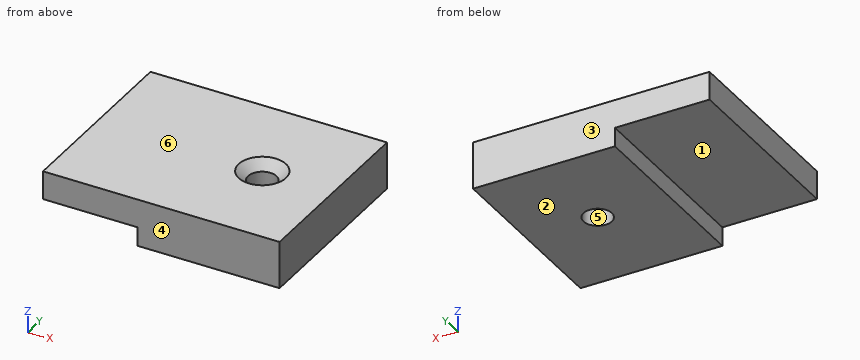
```python
from build123d import *

# Parameters (mm, degrees)
F1_DEPTH = 20
F2_R     = 1.5
F3_DEPTH = 5.001
F4_SIZE  = 1


with BuildPart() as f1:
    # F0 (on Front) → F1 (new body)
    with BuildSketch(Plane.XZ):
        Polygon((-22.628114, -7.176122), (-12.628114, -7.176122), (-12.628114, -9.176122), (2.371886, -9.176122), (2.371886, -4.176122), (-22.628114, -4.176122), align=None)
    extrude(amount=F1_DEPTH)

    # F2 (on face) → F3 (cut, through all)
    with BuildSketch(Plane(origin=(0, 0, -9.176122), x_dir=(1, 0, 0), z_dir=(0, 0, -1))):
        with Locations((-5.128114, 10)):
            Circle(F2_R)
    extrude(amount=-F3_DEPTH, mode=Mode.SUBTRACT)

    # F4
    f4_edges = [f1.edges().sort_by_distance(p)[0] for p in [
        (-6.628114, -10, -4.176122),
    ]]
    chamfer(f4_edges, length=F4_SIZE)


solid = f1.part
```
The model under review builds one solid part; all positions refer to its coordinate system, in mm. Face numbers are marked on the shaded views. A direction names the side the tool comes from. Give positions to 0.01 mm unless a question says otherwise; leave off trailing zeros. Write each loop counter-clockwise with the first axis right and the second up, starting at its lowest first coordinate (ties: lowest second). Pieces come first, ordered by that corner, then holes. Notation, with made-up numbers: M -11,23 L 30,23 A22 ccw 30,38 Z; hole C 85,19 d1. An arc over 180 degrees is marked long. Answer in a Markdown table with one row per item.
Item 1: Draft analysis for pull direction Y (two halves, no side actions). For the marked faces 3, 4, 5 and 6, state which applies: +Y half, -Y half, draft (parallel to the pull), parting line (faces both ways), or undercut.
Check sheet entries:
| item | result |
|---|---|
| face 3 | +Y half |
| face 4 | -Y half |
| face 5 | undercut |
| face 6 | draft |
Item 2: Add section A-A on y = -10. Give the boundary of the cut face in (x, z).
Check sheet entries:
| item | result |
|---|---|
| outline | M -22.63,-7.18 L -12.63,-7.18 L -12.63,-9.18 L -6.63,-9.18 L -6.63,-5.18 L -7.63,-4.18 L -22.63,-4.18 Z; M -3.63,-9.18 L 2.37,-9.18 L 2.37,-4.18 L -2.63,-4.18 L -3.63,-5.18 Z |
Item 3: Add section B-B on y = -4.75. Give the boundary of the cut face in (x, z), plus the area to 3 significant figures.
Check sheet entries:
| item | result |
|---|---|
| outline | M -22.63,-7.18 L -12.63,-7.18 L -12.63,-9.18 L 2.37,-9.18 L 2.37,-4.18 L -22.63,-4.18 Z |
| area | 105 mm2 |
Item 4: Add section D-D on x = -16.25. Give the boundary of the cut face in (y, z).
Check sheet entries:
| item | result |
|---|---|
| outline | M -20,-7.18 L 0,-7.18 L 0,-4.18 L -20,-4.18 Z |
Item 5: Tool access review of the marked faces 1 and 2: name each direction out of +Z, -Z, +X, -X, +Y, -Y from which nothing blocks a thin tool from reaching the whole face with its end or side.
Check sheet entries:
| item | result |
|---|---|
| face 1 | -Z, -X, +Y, -Y |
| face 2 | -Z, +X, -X, +Y, -Y |
Item 6: Add section C-C on z = -4.8. Give the boundary of the cut face in (x, y).
Check sheet entries:
| item | result |
|---|---|
| outline | M -22.63,-20 L 2.37,-20 L 2.37,0 L -22.63,0 Z; hole C -5.13,-10 d3.75 |
Item 7: For P1, Ø0.6, axis at y = -13, z = -8, coming from the -X side; P2, Ø2, axis at x = -17, y = -7.5, coming from the -Z side, all flat-tipped, find the tip position at first contact; note any pin that passes through.
Check sheet entries:
| item | result |
|---|---|
| P1 | x = -12.63 |
| P2 | z = -7.18 |
Item 8: For line 1 along X through (y, z) = (-10, -6.55); line 2 along Y through (x, z) = (-5, -7.9); line 3 along X through (y, z) = (-10, -7.25), list the stretches that pass through material, from the lowest coordinate up.
Check sheet entries:
| item | result |
|---|---|
| line 1 | -22.63 to -6.63, -3.63 to 2.37 |
| line 2 | -20 to -11.49, -8.51 to 0 |
| line 3 | -12.63 to -6.63, -3.63 to 2.37 |
